```python
from build123d import *

# Parameters (mm, degrees)
CUT_EXTRUDE1_DEPTH        = 22.5
CIRPATTERN1_COUNT         = 6
M2X0_4_TAPPED_HOLE1_D     = 1.6
M2X0_4_TAPPED_HOLE1_DEPTH = 7
M2X0_4_TAPPED_HOLE1_TIP   = 0.480688495
M2X0_4_TAPPED_HOLE2_D     = 1.6
M2X0_4_TAPPED_HOLE2_DEPTH = 8.2
M2X0_4_TAPPED_HOLE2_TIP   = 0.480688495


with BuildPart() as part:
    # Sketch1 one side → Revolve3 (revolve)
    with BuildSketch(Plane.XY):
        Polygon((12.75, 0), (16.35, 0), (16.35, 3.5), (15, 3.5), (15, 17.778485378), (5.75, 26), (0, 26), (0, 24.5), (3.084626234, 24.5), (3.425, 5), (4.5, 5), (5.696502575, 23.37174091), (12.75, 17.102504994), align=None)
    revolve(axis=Axis((0, 0, 0), (0, 1, 0)))

    # Sketch2 → Cut-Extrude1 (cut)
    with BuildSketch(Plane(origin=(0, 26, 0), x_dir=(1, 0, 0), z_dir=(0, 1, 0))):
        with BuildLine():
            Line((13.781237245, -4), (14.456832295, -4))
            ThreePointArc((14.456832295, -4), (15, 0), (14.456832295, 4))
            Line((14.456832295, 4), (13.781237245, 4))
            ThreePointArc((13.781237245, 4), (14.35, 0), (13.781237245, -4))
        make_face()
    cut_extrude1 = extrude(amount=-CUT_EXTRUDE1_DEPTH, mode=Mode.SUBTRACT)

    # CirPattern1: Cut-Extrude1 ×6 about axis
    cirpattern1_axis = Axis((0, 0, 0), (0, 1, 0))
    for i in range(1, CIRPATTERN1_COUNT):
        add(cut_extrude1.rotate(cirpattern1_axis, i * 360 / CIRPATTERN1_COUNT), mode=Mode.SUBTRACT)

    # M2x0.4 Tapped Hole1
    with Locations(Plane.XY.offset(16.35)):
        with Locations((0, 1.75)):
            Hole(M2X0_4_TAPPED_HOLE1_D / 2, depth=M2X0_4_TAPPED_HOLE1_DEPTH)
            with Locations((0, 0, -(M2X0_4_TAPPED_HOLE1_DEPTH + M2X0_4_TAPPED_HOLE1_TIP / 2))):  # 118° drill point
                Cone(0, M2X0_4_TAPPED_HOLE1_D / 2, M2X0_4_TAPPED_HOLE1_TIP, mode=Mode.SUBTRACT)

    # M2x0.4 Tapped Hole2
    with Locations(Plane(origin=(0, 0, -16.35), x_dir=(-1, 0, 0), z_dir=(0, 0, -1))):
        with Locations((0, 1.75)):
            Hole(M2X0_4_TAPPED_HOLE2_D / 2, depth=M2X0_4_TAPPED_HOLE2_DEPTH)
            with Locations((0, 0, -(M2X0_4_TAPPED_HOLE2_DEPTH + M2X0_4_TAPPED_HOLE2_TIP / 2))):  # 118° drill point
                Cone(0, M2X0_4_TAPPED_HOLE2_D / 2, M2X0_4_TAPPED_HOLE2_TIP, mode=Mode.SUBTRACT)


solid = part.part
```
Model file for the job. Use its own axes, mm. A direction names the side the tool comes from. Coordinates: 2 decimals unless noted, no trailing zeros. Loops run counter-clockwise (first coordinate to the right, second up) from the corner with the lowest first, then second, coordinate; pieces in that order, holes last. Notation, with made-up numbers: (49, 75.25) - (69, 75.25) arc R7 ccw to (69, 79.25) - close; hole circle Ø4 at (70.25, 15.25). An arc over 180 degrees is marked (long way). Answer as a JSON object with one key per item and string values. Group by question number.
(1) Probe line 1 along X through (y, z) = (8.75, 0); line 2 along Z through (x, y) = (0.5, 19.5); line 3 along Z through (x, y) = (-4, 19.5). List the from-to ranges inside material, lowest first.
(2) Cut at B-B (x = 0). State how many separate pieces and enclosed holes the cut face has, then the cut area to 3 significant figures.
(3) Cut at A-A (y = 11.75). Give the cut face in (x, z), then the cut area to 3 significant figures.
(4) Cut at D-D (y = 15.5). Give the cut face in (x, z), then the cut area to 3 significant figures.
(5) Two-plate mould, pull along X, no slides. Class faces 4 (the face through (-12.96, 10.74, -7.55)), 5 (the face through (0, 11, -15)), 6 (the face through (3, 5, 2)): released by +X, released by -X, zero draft, split by the parting line, or undercut.
(6) Tool access for faces 1 (the face through (-0.71, 14.61, 3.18)), 2 (the face through (12.96, 10.74, 7.55)), 3 (the face through (13.02, 10.74, -7.45)): list every direction of +Z, -Z, +X, -X, +Y, -Y with a clear straight run to the whole face (end or side of a thin tool).
(7) Flat gauge pins, fed straight in: pin 1 (4 mm diameter, centred on x = 2.5, z = -13, fed in from +Y); pin 2 (3 mm diameter, centred on x = -11, y = 10.5, fed in from +Z); pin 3 (6 mm diameter, centred on x = -9, y = 8.5, fed in from +Z). Where does each tip first touch, or does it go through?
Geometry says:
{
 "1": {"line 1": "x = -14.35 to -12.75, -4.74 to -3.36, 3.36 to 4.74, 12.75 to 14.35", "line 2": "z = -13.05 to -10.04, -5.42 to -3.13, 3.13 to 5.42, 10.04 to 13.05", "line 3": "z = -12.44 to -9.22, -3.69 to 3.69, 9.22 to 12.44"},
 "2": {"separate pieces": "3", "enclosed holes": "0", "area": "211 mm^2"},
 "3": {"outline": "(-14.46, -4) arc R15 ccw to (-10.69, -10.52) - (-10.35, -9.93) arc R14.35 ccw to (-3.43, -13.93) - (-3.76, -14.52) arc R15 ccw to (3.76, -14.52) - (3.43, -13.93) arc R14.35 ccw to (10.35, -9.93) - (10.69, -10.52) arc R15 ccw to (14.46, -4) - (13.78, -4) arc R14.35 ccw to (13.78, 4) - (14.46, 4) arc R15 ccw to (10.69, 10.52) - (10.35, 9.93) arc R14.35 ccw to (3.43, 13.93) - (3.76, 14.52) arc R15 ccw to (-3.76, 14.52) - (-3.43, 13.93) arc R14.35 ccw to (-10.35, 9.93) - (-10.69, 10.52) arc R15 ccw to (-14.46, 4) - (-13.78, 4) arc R14.35 ccw to (-13.78, -4) - close; circle Ø9.88 at (0, 0); hole circle Ø25.5 at (0, 0); hole circle Ø6.61 at (0, 0)", "area": "207 mm^2"},
 "4": {"outline": "(-14.46, -4) arc R15 ccw to (-10.69, -10.52) - (-10.35, -9.93) arc R14.35 ccw to (-3.43, -13.93) - (-3.76, -14.52) arc R15 ccw to (3.76, -14.52) - (3.43, -13.93) arc R14.35 ccw to (10.35, -9.93) - (10.69, -10.52) arc R15 ccw to (14.46, -4) - (13.78, -4) arc R14.35 ccw to (13.78, 4) - (14.46, 4) arc R15 ccw to (10.69, 10.52) - (10.35, 9.93) arc R14.35 ccw to (3.43, 13.93) - (3.76, 14.52) arc R15 ccw to (-3.76, 14.52) - (-3.43, 13.93) arc R14.35 ccw to (-10.35, 9.93) - (-10.69, 10.52) arc R15 ccw to (-14.46, 4) - (-13.78, 4) arc R14.35 ccw to (-13.78, -4) - close; circle Ø10.37 at (0, 0); hole circle Ø25.5 at (0, 0); hole circle Ø6.48 at (0, 0)", "area": "216 mm^2"},
 "5": {"face 4": "released by -X", "face 5": "split by the parting line", "face 6": "undercut"},
 "6": {"face 1": "-Y", "face 2": "+Z, +X, +Y", "face 3": "-Z, +X, +Y"},
 "7": {"pin 1": "stops at y = 21.12", "pin 2": "stops at z = 10.76", "pin 3": "stops at z = 13.04"}
}
